Work out the finished part from the listing and answer in its coordinate system (mm). A direction names the side the tool comes from. Round coordinates to 2 decimals unless told otherwise and drop trailing zeros. Order: outer loops, then holes, each group sorted by start corner. A loop starts at its lowest first (then second) coordinate and runs counter-clockwise, first axis right, second up.
from build123d import *

# Parameters (mm, degrees)
FILLET2_R = 1.27
FILLET3_R = 0.635


with BuildPart() as part:
    # Sketch1 → Revolve4 (revolve)
    with BuildSketch(Plane.XY):
        Polygon((12.334639896, 0), (21.75, 0), (21.75, 3), (25, 3), (25, 6.25), (18.035610483, 6.25), (18.035610483, 28.23587128), (13.370385965, 28.23587128), (13.370385965, 36.611095198), (2.974741934, 36.611095198), (2.974741934, 28.23587128), (0, 28.23587128), (0, 25.3), (2.830568931, 25.3), (2.974741934, 25.3), (12.334639896, 25.3), align=None)
    revolve(axis=Axis((0, 0, 0), (0, 1, 0)))

    # Fillet2
    fillet2_edges = [part.edges().sort_by_distance(p)[0] for p in [
        (-13.370385965, 28.23587128, 0),
        (-18.035610483, 6.25, 0),
    ]]
    fillet(fillet2_edges, radius=FILLET2_R)

    # Fillet3
    fillet3_edges = [part.edges().sort_by_distance(p)[0] for p in [
        (-13.370385965, 36.611095198, 0),
    ]]
    fillet(fillet3_edges, radius=FILLET3_R)


solid = part.part
Item 1: Given pin 1 (3.5 mm diameter, centred on x = 0, z = 0, fed in from -Y); pin 2 (1 mm diameter, centred on x = 0, z = -2, fed in from +Y); pin 3 (4 mm diameter, centred on y = 18, z = -2, fed in from -X), each flat-ended and moving along its own axis, determine where each tip first touches the part or whether it passes through.
Item 2: Find section B-B (y = 11.5). Write down the section's boundary in (x, z).
Item 3: Find section D-D (y = 26). Write down the section's boundary in (x, z).
Item 4: Find the intervals of material crossed by line 1 along Z through (x, y) = (0, 15.25); line 2 along X through (y, z) = (30.25, 0), in increasing order.
Item 5: A tool of negligible diameter and unlimited length cuts with its end or side. For faces 1 (the face through (0, 25.3, 0)), 2 (the face through (0, 28.236, 0)), 3 (the face through (3, 36.611, 3)), from which of +Z, -Z, +X, -X, +Y, -Y can it reach the whole face along a straight path? Write none if from no direction.
Model answer:
1. pin 1: stops at y = 25.3
1. pin 2: stops at y = 28.24
1. pin 3: stops at x = -18.04
2. outline: circle Ø36.07 at (0, 0); hole circle Ø24.67 at (0, 0)
3. outline: circle Ø36.07 at (0, 0)
4. line 1: z = -18.04 to -12.33, 12.33 to 18.04
4. line 2: x = -13.37 to -2.97, 2.97 to 13.37
5. face 1: -Y
5. face 2: +Y
5. face 3: +Z, -Z, +X, -X, +Y
